Job drawing, mm, ordinate dimensions from the low corner. One solid piece. Give positions to 0.01 mm unless a question says otherwise; leave off trailing zeros. Write each loop counter-clockwise with the first axis right and the second up, starting at its lowest first coordinate (ties: lowest second). Pieces come first, ordered by that corner, then holes. Notation, with made-up numbers: (81.25, -12.75) - (99.25, -12.75) arc R8 cw to (99.25, 1.25) - close; hole circle Ø6 at (7, -37.5). An arc over 180 degrees is marked (long way). Answer in a Markdown table with one row per item. Add a question column.
1. Band-saw the part on A-A on x = 89.85. Write the cut outline in (y, z), plus the area to 3 significant figures.
2. Band-saw the part on B-B on y = 12.5. Write the cut outline in (x, z), plus the area to 3 significant figures.
3. Probe line 1 along X through (y, z) = (12.5, 2.55); line 2 along X through (y, z) = (12.5, 0.65); line 3 along Y through (x, z) = (89.85, 2.4). List the from-to ranges inside material, lowest first.
4. Drop flat-ended pins along their axis: pin 1 Ø6.5 at (x, y) = (6.35, 12.5) entering from -Z; pin 2 Ø4.5 at (x, y) = (89.85, 12.5) entering from +Z. Give the stop position or say it passes through.
5. Band-saw the part on C-C on z = 4.15. Write the cut outline in (x, y).
6. Band-saw the part on D-D on x = 133.35. Write the cut outline in (y, z).
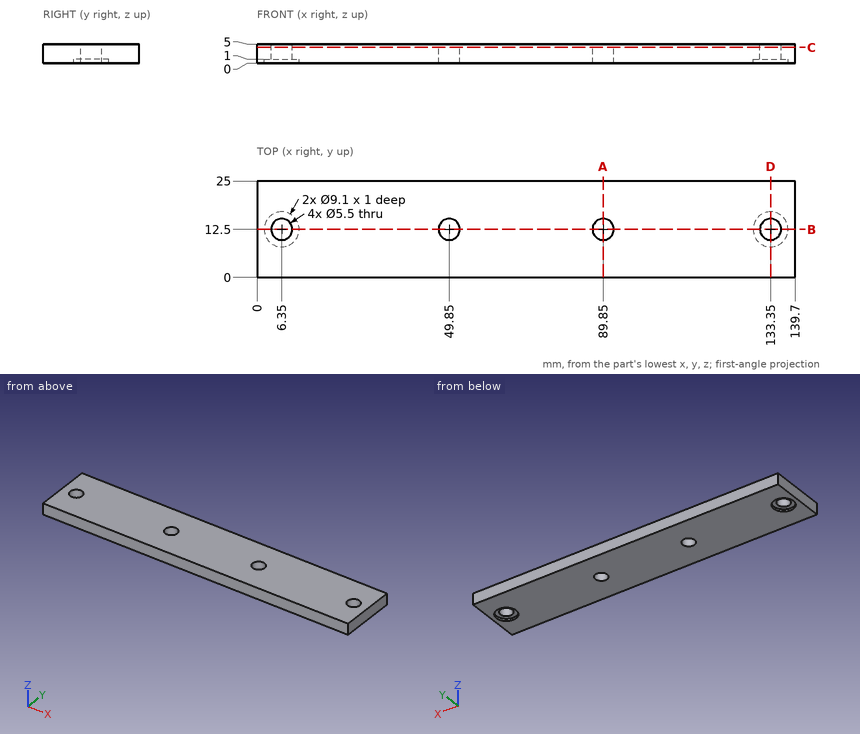
Values:
| question | item | result |
|---|---|---|
| 1 | outline | (0, 0) - (9.75, 0) - (9.75, 5) - (0, 5) - close; (15.25, 0) - (25, 0) - (25, 5) - (15.25, 5) - close |
| 1 | area | 97.5 mm² |
| 2 | outline | (0, 0) - (1.8, 0) - (1.8, 1) - (3.6, 1) - (3.6, 5) - (0, 5) - close; (9.1, 1) - (10.9, 1) - (10.9, 0) - (47.1, 0) - (47.1, 5) - (9.1, 5) - close; (52.6, 0) - (87.1, 0) - (87.1, 5) - (52.6, 5) - close; (92.6, 0) - (128.8, 0) - (128.8, 1) - (130.6, 1) - (130.6, 5) - (92.6, 5) - close; (136.1, 1) - (137.9, 1) - (137.9, 0) - (139.7, 0) - (139.7, 5) - (136.1, 5) - close |
| 2 | area | 581 mm² |
| 3 | line 1 | x = 0 to 3.6, 9.1 to 47.1, 52.6 to 87.1, 92.6 to 130.6, 136.1 to 139.7 |
| 3 | line 2 | x = 0 to 1.8, 10.9 to 47.1, 52.6 to 87.1, 92.6 to 128.8, 137.9 to 139.7 |
| 3 | line 3 | y = 0 to 9.75, 15.25 to 25 |
| 4 | pin 1 | stops at z = 1 |
| 4 | pin 2 | passes through |
| 5 | outline | (0, 0) - (139.7, 0) - (139.7, 25) - (0, 25) - close; hole circle Ø5.5 at (6.35, 12.5); hole circle Ø5.5 at (49.85, 12.5); hole circle Ø5.5 at (89.85, 12.5); hole circle Ø5.5 at (133.35, 12.5) |
| 6 | outline | (0, 0) - (7.95, 0) - (7.95, 1) - (9.75, 1) - (9.75, 5) - (0, 5) - close; (15.25, 1) - (17.05, 1) - (17.05, 0) - (25, 0) - (25, 5) - (15.25, 5) - close |
